```python
from build123d import *

# Parameters (mm, degrees)
SKETCH1_W                     = 88.9
SKETCH1_H                     = 12.7
SMALL_BASE_EXTRUDE_DEPTH      = 5.08
SKETCH3_W                     = 30.48
SKETCH3_H                     = 12.7
MAIN_TOWER_EXTRUDE_DEPTH      = 121.92
SKETCH4_W                     = 12.7
SKETCH4_H                     = 107.95
FILAMENT_CHANNEL_CUT_DEPTH    = 13.7
SKETCH6_R                     = 2.03962
CUT_EXTRUDE3_DEPTH            = 8.89
LPATTERN1_COUNT               = 4
LPATTERN1_PITCH               = 34.29
SKETCH9_R                     = 2.03962
CUT_EXTRUDE6_DEPTH            = 8.89
LPATTERN2_COUNT               = 4
LPATTERN2_PITCH               = 34.29
SKETCH10_W                    = 5.08
SKETCH10_H                    = 3.2766
WIRE_CHANNEL_CUT_DEPTH        = 228.6
SKETCH11_R                    = 3.175
MOUNTING_BOLT_HOLE_CUTS_DEPTH = 25.4
COPPER_BOARD_EXTRUDE_DEPTH    = 80.16
SKETCH13_W                    = 30.48
SKETCH13_H                    = 64.772627344
COPPER_BOARD_CUT_DEPTH        = 10.16
WIRE_ESCAPE_HOLE_CUT_DEPTH    = 5.08


with BuildPart() as part:
    # Sketch1 → Small Base Extrude (new body)
    with BuildSketch(Plane(origin=(0, 0, 0), x_dir=(1, 0, 0), z_dir=(0, 0, -1))):
        with Locations((0, -6.35)):
            Rectangle(SKETCH1_W, SKETCH1_H)
    extrude(amount=SMALL_BASE_EXTRUDE_DEPTH)

    # Sketch3 → Main Tower Extrude (add)
    with BuildSketch(Plane(origin=(0, 0, -5.08), x_dir=(1, 0, 0), z_dir=(0, 0, -1))):
        with Locations((0, -6.35)):
            Rectangle(SKETCH3_W, SKETCH3_H)
    extrude(amount=MAIN_TOWER_EXTRUDE_DEPTH)

    # Sketch4 → Filament Channel Cut (cut, through all)
    with BuildSketch(Plane(origin=(0, 12.7, 0), x_dir=(1, 0, 0), z_dir=(0, 1, 0))):
        with Locations((0, 64.135)):
            Rectangle(SKETCH4_W, SKETCH4_H)
    extrude(amount=-FILAMENT_CHANNEL_CUT_DEPTH, mode=Mode.SUBTRACT)

    # Sketch6 → Cut-Extrude3 (cut)
    with BuildSketch(Plane(origin=(-6.35, 0, 0), x_dir=(0, 0, -1), z_dir=(1, 0, 0))):
        with Locations((12.7, 6.35)):
            Circle(SKETCH6_R)
    cut_extrude3 = extrude(amount=-CUT_EXTRUDE3_DEPTH, mode=Mode.SUBTRACT)

    # LPattern1: Cut-Extrude3 ×4
    with Locations(*[(0, 0, -i * LPATTERN1_PITCH) for i in range(1, LPATTERN1_COUNT)]):
        add(cut_extrude3, mode=Mode.SUBTRACT)

    # Sketch9 → Cut-Extrude6 (cut)
    with BuildSketch(Plane(origin=(6.35, 57.001874069, -16.025022356), x_dir=(0, 0, 1), z_dir=(-1, 0, 0))):
        with Locations((3.325022356, -50.651874069)):
            Circle(SKETCH9_R)
    cut_extrude6 = extrude(amount=-CUT_EXTRUDE6_DEPTH, mode=Mode.SUBTRACT)

    # LPattern2: Cut-Extrude6 ×4
    with Locations(*[(0, 0, -i * LPATTERN2_PITCH) for i in range(1, LPATTERN2_COUNT)]):
        add(cut_extrude6, mode=Mode.SUBTRACT)

    # Sketch10 → Wire Channel Cut (cut)
    with BuildSketch(Plane(origin=(0, 0, -127), x_dir=(-1, 0, 0), z_dir=(0, 0, -1))):
        with Locations((12.7, 6.35)):
            Rectangle(SKETCH10_W, SKETCH10_H)
        with Locations((-12.7, 6.35)):
            Rectangle(SKETCH10_W, SKETCH10_H)
    extrude(amount=-WIRE_CHANNEL_CUT_DEPTH, mode=Mode.SUBTRACT)

    # Sketch11 → Mounting Bolt Hole Cuts (cut)
    with BuildSketch(Plane.XY):
        with Locations((38.1, 6.35)):
            Circle(SKETCH11_R)
        with Locations((-38.1, 6.35)):
            Circle(SKETCH11_R)
    extrude(amount=-MOUNTING_BOLT_HOLE_CUTS_DEPTH, mode=Mode.SUBTRACT)

    # Sketch12 → Copper Board Extrude (add)
    with BuildSketch(Plane(origin=(0, 12.7, 0), x_dir=(1, 0, 0), z_dir=(0, 1, 0))):
        Polygon((-15.24, 0), (15.24, 0), (20.32, 0), (20.32, 5.08), (15.24, 5.08), (15.24, 10.16), (-15.24, 10.16), (-15.24, 5.08), (-20.32, 5.08), (-20.32, 0), align=None)
    extrude(amount=COPPER_BOARD_EXTRUDE_DEPTH)

    # Sketch13 → Copper Board Cut (cut)
    with BuildSketch(Plane(origin=(0, 0, -10.16), x_dir=(-1, 0, 0), z_dir=(0, 0, -1))):
        with Locations((0, 50.166313672)):
            Rectangle(SKETCH13_W, SKETCH13_H)
    extrude(amount=-COPPER_BOARD_CUT_DEPTH, mode=Mode.SUBTRACT)

    # Sketch14 → Wire Escape Hole Cut (cut)
    with BuildSketch(Plane.XY):
        Polygon((-10.16, 4.7117), (10.16, 4.7117), (10.16, 7.9883), (10.16, 17.78), (-10.16, 17.78), (-10.16, 6.0833), align=None)
    extrude(amount=-WIRE_ESCAPE_HOLE_CUT_DEPTH, mode=Mode.SUBTRACT)


solid = part.part
```
The listing builds one solid part. Answer for the finished solid, in the listing's coordinates (mm). A direction names the side the tool comes from. Give positions to 0.01 mm unless a question says otherwise; leave off trailing zeros. Write each loop counter-clockwise with the first axis right and the second up, starting at its lowest first coordinate (ties: lowest second). Pieces come first, ordered by that corner, then holes. Notation, with made-up numbers: (-10, -17.5) -> (7, -17.5) arc R33 ccw to (7, 18.5) -> close; hole circle Ø11 at (59.5, 51.25). An arc over 180 degrees is marked (long way). Use one line per item in the form item = value.
1) Each of these flat-tipped pins is pushed along its axis until it touches: P1, Ø4.5, axis at y = 6.35, z = -12.7, coming from the +X side; P2, Ø3.5, axis at y = 6.5, z = -120, coming from the -X side; P3, Ø2.5, axis at x = 12.5, z = -123.5, coming from the +Y side. Where does it stop, or does it pass through?
Result:
P1 = 15.24
P2 = -15.24
P3 = 12.7
2) Section B-B on x = -12 is taken. Count the separate pieces of the cut face and the enclosed holes in it, plus the area to 3 significant figures.
Result:
separate_pieces = 3
enclosed_holes = 0
area = 1,350 mm²
3) Section D-D on x = 38.1 is taken. Write down the section's boundary in (y, z) (3 decimals), plus the area to 3 significant figures.
Result:
outline = (0, -5.08) -> (3.175, -5.08) -> (3.175, 0) -> (0, 0) -> close; (9.525, -5.08) -> (12.7, -5.08) -> (12.7, 0) -> (9.525, 0) -> close
area = 32.3 mm²
4) For a pull along Z with two mould halves and no side action, classify faces 5 (the flat face through (13, 7.988, -6)), 6 (the cylindrical face through (-9.745, 6.963, -14.645)), 7 (the flat face through (-20, 29, -5.08)) as +Z half, -Z half, draft (parallel to the pull), parting line (faces both ways), or undercut.
Result:
face_5 = draft
face_6 = undercut
face_7 = -Z half
5) Section C-C on y = 43 is taken. Write down the section's boundary in (x, z).
Result:
outline = (-20.32, -5.08) -> (-15.24, -5.08) -> (-15.24, 0) -> (-20.32, 0) -> close; (15.24, -5.08) -> (20.32, -5.08) -> (20.32, 0) -> (15.24, 0) -> close
6) A tool of negligible diameter and unlimited length cuts with its end or side. For faces 1 (the flat face through (-15.24, 10, -67)), 2 (the flat face through (13, 7.988, -30)), 3 (the flat face through (15.24, 2, -65)), 4 (the flat face through (15.24, 6, -3)), from which of +Z, -Z, +X, -X, +Y, -Y can it reach the whole face along a straight path? Write none if from no direction.
Result:
face_1 = -Z, -X, +Y, -Y
face_2 = +Z, -Z, +X
face_3 = -Z, +X, +Y, -Y
face_4 = +Z, -Z
7) Straight lines are drawn through the part: probe 1 along Y at (x, z) = (-12.5, -9); probe 2 along Z at (x, y) = (-4, 8.5); probe 3 along Y at (x, z) = (12.75, -12.7). For each, find the intervals that lie inside material, in ascending order.
Result:
probe_1 = 0 to 4.71, 7.99 to 17.78, 82.55 to 92.86
probe_2 = -127 to -118.11, -10.16 to -5.08
probe_3 = 0 to 4.31, 8.39 to 12.7
8) Section A-A on z = -106 is taken. Write down the section's boundary in (x, y), plus the area to 3 significant figures.
Result:
outline = (-15.24, 0) -> (-6.35, 0) -> (-6.35, 12.7) -> (-15.24, 12.7) -> (-15.24, 7.99) -> (-10.16, 7.99) -> (-10.16, 4.71) -> (-15.24, 4.71) -> close; (6.35, 0) -> (15.24, 0) -> (15.24, 4.71) -> (10.16, 4.71) -> (10.16, 7.99) -> (15.24, 7.99) -> (15.24, 12.7) -> (6.35, 12.7) -> close
area = 193 mm²
